Geometry check sheet. Reference: drawing and pictorial views, mm from the part's lowest x, y, z. A direction names the side the tool comes from. Coordinates: 2 decimals unless noted, no trailing zeros. Loops run counter-clockwise (first coordinate to the right, second up) from the corner with the lowest first, then second, coordinate; pieces in that order, holes last. Notation, with made-up numbers: (-30.5, 13.5) - (5.5, 13.5) arc R21 cw to (5.5, 47.5) - close; hole circle Ø7 at (43, 61.5). An arc over 180 degrees is marked (long way). One line per item, written item: value.
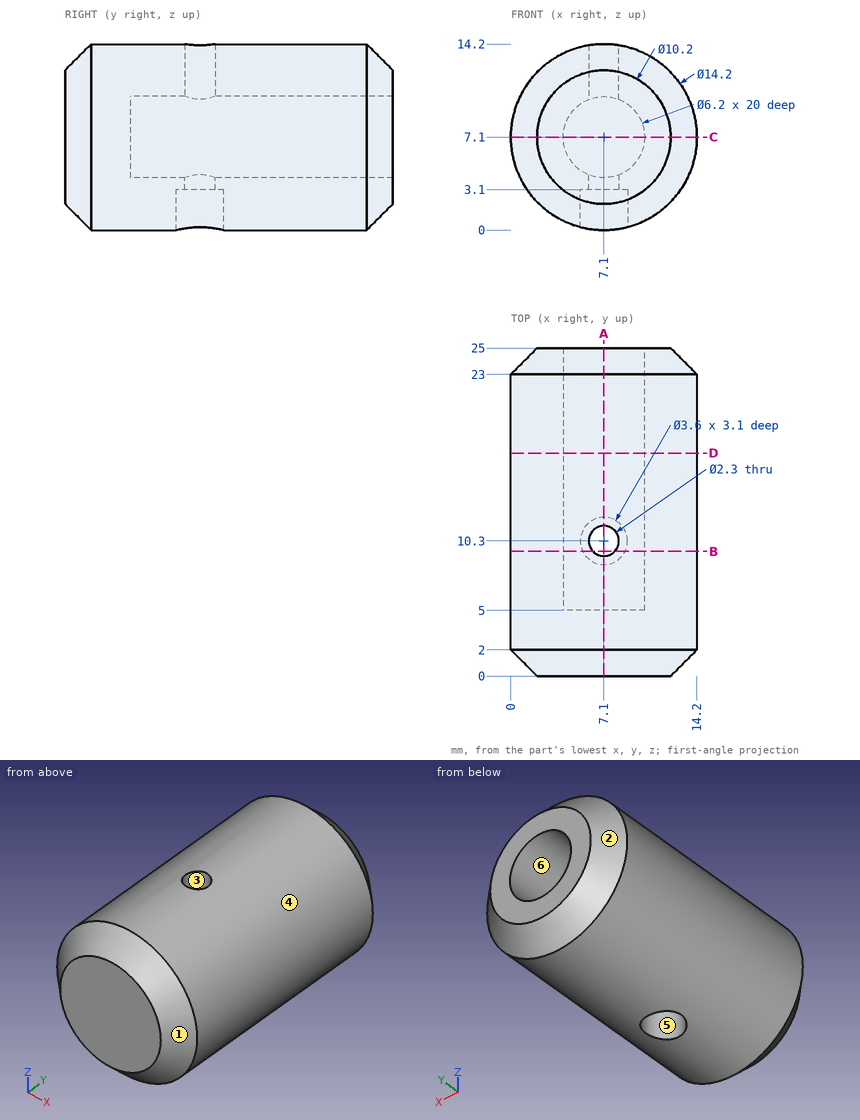
(1) Cross-section at B-B on y = 9.5. Record the cut outline in (x, z).
Reply:
outline: (5.49, 0.19) - (5.49, 3.1) - (6.27, 3.1) - (6.27, 4.11) arc R3.1 cw to (6.27, 10.09) - (6.27, 14.15) arc R7.1 ccw to start; (7.93, 3.1) - (8.71, 3.1) - (8.71, 0.19) arc R7.1 ccw to (7.93, 14.15) - (7.93, 10.09) arc R3.1 cw to (7.93, 4.11) - close
(2) Go/stop test with flat-tipped pins: pin 1 Ø1.9 at (x, z) = (5.5, 7.5) entering from +Y; pin 2 Ø1 at (y, z) = (11, 3.5) entering from +X; pin 3 Ø5 at (y, z) = (10, 12.5) entering from -X. Record where each tip stops, or that it passes through.
Reply:
pin 1: y = 5
pin 2: x = 13.49
pin 3: x = 0.62
(3) Material ranges on probe 1 along Y at (x, z) = (7.1, 3.5); probe 2 along Z at (x, y) = (7.1, 13); probe 3 along Y at (x, z) = (5.25, 8.5), recorded low to high. Write a range as from..to.
Reply:
probe 1: 0..9.15, 11.45..25
probe 2: 0..4, 10.2..14.2
probe 3: 0..5
(4) Cross-section at D-D on y = 17. Record the cut outline in (x, z).
Reply:
outline: circle Ø14.2 at (7.1, 7.1); hole circle Ø6.2 at (7.1, 7.1)
(5) Release check for a two-part mould opening along Y. For the marked faces 1, 2 and 3 record: pulls with the +Y half, pulls with the -Y half, needs draft (parallel to the pull), parting line crosses it, or undercut.
Reply:
face 1: pulls with the -Y half
face 2: pulls with the +Y half
face 3: undercut
(6) Cross-section at C-C on z = 7.1. Record the cut outline in (x, y), and give its area (3 significant figures).
Reply:
outline: (0, 2) - (2, 0) - (12.2, 0) - (14.2, 2) - (14.2, 23) - (12.2, 25) - (10.2, 25) - (10.2, 5) - (4, 5) - (4, 25) - (2, 25) - (0, 23) - close
area: 223 mm2
(7) Access from +Z, -Z, +X, -X, +Y, -Y to the whole of each face (thin tool, end or side, straight path). Record for the marked faces 4, 5 and 6.
Reply:
face 4: +Y, -Y
face 5: -Z
face 6: +Y
(8) Cross-section at A-A on x = 7.1. Record the cut outline in (y, z).
Reply:
outline: (0, 2) - (2, 0) - (8.5, 0) - (8.5, 3.1) - (9.15, 3.1) - (9.15, 4) - (5, 4) - (5, 10.2) - (9.15, 10.2) - (9.15, 14.2) - (2, 14.2) - (0, 12.2) - close; (11.45, 3.1) - (12.1, 3.1) - (12.1, 0) - (23, 0) - (25, 2) - (25, 4) - (11.45, 4) - close; (11.45, 10.2) - (25, 10.2) - (25, 12.2) - (23, 14.2) - (11.45, 14.2) - close
